Could you check a few things on this model? Use its own coordinates, in mm. Face numbers are marked on the shaded views. A direction names the side the tool comes from. Give positions to 0.01 mm unless a question says otherwise; leave off trailing zeros. Loops run counter-clockwise (first coordinate to the right, second up) from the corner with the lowest first, then second, coordinate; pieces in that order, holes last. Notation, with made-up numbers: M 60.25,54.5 L 65.25,54.5 A31 cw 65.25,88.5 Z; hole C -35,-33.75 d5. An arc over 180 degrees is marked long. Answer in a Markdown table with one row per item. Add a question column.
1. Which directions (+Z, -Z, +X, -X, +Y, -Y) give clear straight access to the entire face, cutting with the end or side of a thin tool? Please do the marked faces 3, 4, 5 and 6.
2. If we section it at D-D on y = -7.5: List the corners of the cut face in (x, z) for me.
3. Thinking about a two-plate mould opening in X: for the marked faces 1 and 2, which applies, released by +X, released by -X, zero draft, split by the parting line, or undercut?
4. I need wall thicknesses on line 1 along Y through (x, z) = (0, 11); line 2 along X through (y, z) = (19, 3.75); line 3 along X through (y, z) = (22.5, 10). Which ranges of each line are inside material? Lowest first, please. Write a range as from..to.
5. I'm going to push flat-ended pins straight in: pin 1 Ø2 at (y, z) = (-10, 11.5) entering from -X; pin 2 Ø4.5 at (x, y) = (-10.11, -10.45) entering from +Z; pin 3 Ø0.8 at (x, y) = (33, 0) entering from -Z. Where does each tip first touch, or does it pass through?
6. If we section it at A-A on z = 14.5: List the corners of the cut face in (x, y) for me, then the cut area to 3 significant figures.
7. If we section it at B-B on y = 0: Count the separate pieces of the cut face and the enclosed holes in it, then the cut area to 3 significant figures.
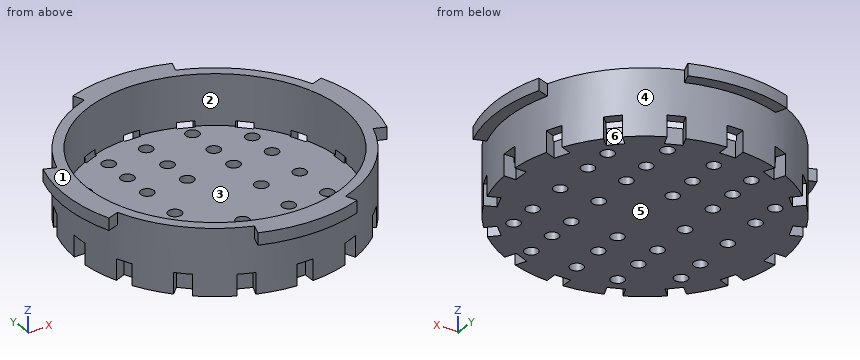
```python
from build123d import *

# Parameters (mm, degrees)
F0_R     = 34.25
F0_R_2   = 31.75
F1_DEPTH = 16.5
F2_R     = 34.25
F2_R_2   = 31.75
F3_DEPTH = 4
F5_DEPTH = 5.25
F7_D     = 3.3
F9_DEPTH = 3


with BuildPart() as f1:
    # F0 (on Top) → F1 (new body)
    with BuildSketch(Plane.XY):
        Circle(F0_R)
        Circle(F0_R_2, mode=Mode.SUBTRACT)
    extrude(amount=F1_DEPTH)

    # F2 (on face) → F3 (join)
    with BuildSketch(Plane(origin=(0, 0, 0), x_dir=(1, 0, 0), z_dir=(0, 0, -1))):
        Circle(F2_R)
        Circle(F2_R_2, mode=Mode.SUBTRACT)
        Circle(F2_R_2)
    extrude(amount=-F3_DEPTH)

    # F4 (on face) → F5 (cut)
    with BuildSketch(Plane(origin=(0, 0, 0), x_dir=(1, 0, 0), z_dir=(0, 0, -1))):
        with BuildLine():
            ThreePointArc((25.5912946517, 22.762867527), (24.2184072556, 24.2184072556), (22.762867527, 25.5912946517))
            Line((22.762867527, 25.5912946517), (20.6828733497, 23.5113004745))
            Line((20.6828733497, 23.5113004745), (23.5113004745, 20.6828733497))
            Line((23.5113004745, 20.6828733497), (25.5912946517, 22.762867527))
        make_face()
        with BuildLine():
            ThreePointArc((14.9323010635, 30.8235118854), (13.1069075585, 31.6428739885), (11.2367829334, 32.3542456149))
            Line((11.2367829334, 32.3542456149), (10.1110981964, 29.6366022557))
            Line((10.1110981964, 29.6366022557), (13.8066163264, 28.1058685262))
            Line((13.8066163264, 28.1058685262), (14.9323010635, 30.8235118854))
        make_face()
        with BuildLine():
            ThreePointArc((2, 34.1915559751), (0, 34.25), (-2, 34.1915559751))
            Line((-2, 34.1915559751), (-2, 31.25))
            Line((-2, 31.25), (2, 31.25))
            Line((2, 31.25), (2, 34.1915559751))
        make_face()
        with BuildLine():
            Line((-10.1110981964, 29.6366022557), (-11.2367829334, 32.3542456149))
            ThreePointArc((-11.2367829334, 32.3542456149), (-13.1069075585, 31.6428739885), (-14.9323010635, 30.8235118854))
            Line((-14.9323010635, 30.8235118854), (-13.8066163264, 28.1058685262))
            Line((-13.8066163264, 28.1058685262), (-10.1110981964, 29.6366022557))
        make_face()
        with BuildLine():
            Line((-20.6828733497, 23.5113004745), (-22.762867527, 25.5912946517))
            ThreePointArc((-22.762867527, 25.5912946517), (-24.2184072556, 24.2184072556), (-25.5912946517, 22.762867527))
            Line((-25.5912946517, 22.762867527), (-23.5113004745, 20.6828733497))
            Line((-23.5113004745, 20.6828733497), (-20.6828733497, 23.5113004745))
        make_face()
        with BuildLine():
            Line((-31.25, 2), (-34.1915559751, 2))
            ThreePointArc((-34.1915559751, 2), (-34.25, 0), (-34.1915559751, -2))
            Line((-34.1915559751, -2), (-31.25, -2))
            Line((-31.25, -2), (-31.25, 2))
        make_face()
        with BuildLine():
            Line((-29.6366022557, -10.1110981964), (-32.3542456149, -11.2367829334))
            ThreePointArc((-32.3542456149, -11.2367829334), (-31.6428739885, -13.1069075585), (-30.8235118854, -14.9323010635))
            Line((-30.8235118854, -14.9323010635), (-28.1058685262, -13.8066163264))
            Line((-28.1058685262, -13.8066163264), (-29.6366022557, -10.1110981964))
        make_face()
        with BuildLine():
            Line((-23.5113004745, -20.6828733497), (-25.5912946517, -22.762867527))
            ThreePointArc((-25.5912946517, -22.762867527), (-24.2184072556, -24.2184072556), (-22.762867527, -25.5912946517))
            Line((-22.762867527, -25.5912946517), (-20.6828733497, -23.5113004745))
            Line((-20.6828733497, -23.5113004745), (-23.5113004745, -20.6828733497))
        make_face()
        with BuildLine():
            Line((-13.8066163264, -28.1058685262), (-14.9323010635, -30.8235118854))
            ThreePointArc((-14.9323010635, -30.8235118854), (-13.1069075585, -31.6428739885), (-11.2367829334, -32.3542456149))
            Line((-11.2367829334, -32.3542456149), (-10.1110981964, -29.6366022557))
            Line((-10.1110981964, -29.6366022557), (-13.8066163264, -28.1058685262))
        make_face()
        with BuildLine():
            Line((-2, -31.25), (-2, -34.1915559751))
            ThreePointArc((-2, -34.1915559751), (0, -34.25), (2, -34.1915559751))
            Line((2, -34.1915559751), (2, -31.25))
            Line((2, -31.25), (-2, -31.25))
        make_face()
        with BuildLine():
            ThreePointArc((11.2367829334, -32.3542456149), (13.1069075585, -31.6428739885), (14.9323010635, -30.8235118854))
            Line((14.9323010635, -30.8235118854), (13.8066163264, -28.1058685262))
            Line((13.8066163264, -28.1058685262), (10.1110981964, -29.6366022557))
            Line((10.1110981964, -29.6366022557), (11.2367829334, -32.3542456149))
        make_face()
        with BuildLine():
            ThreePointArc((30.8235118854, -14.9323010635), (31.6428739885, -13.1069075585), (32.3542456149, -11.2367829334))
            Line((32.3542456149, -11.2367829334), (29.6366022557, -10.1110981964))
            Line((29.6366022557, -10.1110981964), (28.1058685262, -13.8066163264))
            Line((28.1058685262, -13.8066163264), (30.8235118854, -14.9323010635))
        make_face()
        with BuildLine():
            ThreePointArc((22.762867527, -25.5912946517), (24.2184072556, -24.2184072556), (25.5912946517, -22.762867527))
            Line((25.5912946517, -22.762867527), (23.5113004745, -20.6828733497))
            Line((23.5113004745, -20.6828733497), (20.6828733497, -23.5113004745))
            Line((20.6828733497, -23.5113004745), (22.762867527, -25.5912946517))
        make_face()
        with BuildLine():
            ThreePointArc((34.25, 0), (34.2353858759, 1.0004268719), (34.1915559751, 2))
            Line((34.1915559751, 2), (31.25, 2))
            Line((31.25, 2), (31.25, -2))
            Line((31.25, -2), (34.1915559751, -2))
            ThreePointArc((34.1915559751, -2), (34.2353858759, -1.0004268719), (34.25, 0))
        make_face()
        with BuildLine():
            ThreePointArc((32.3542456149, 11.2367829334), (31.6428739885, 13.1069075585), (30.8235118854, 14.9323010635))
            Line((30.8235118854, 14.9323010635), (28.1058685262, 13.8066163264))
            Line((28.1058685262, 13.8066163264), (29.6366022557, 10.1110981964))
            Line((29.6366022557, 10.1110981964), (32.3542456149, 11.2367829334))
        make_face()
        with BuildLine():
            Line((-28.1058685262, 13.8066163264), (-30.8235118854, 14.9323010635))
            ThreePointArc((-30.8235118854, 14.9323010635), (-31.6428739885, 13.1069075585), (-32.3542456149, 11.2367829334))
            Line((-32.3542456149, 11.2367829334), (-29.6366022557, 10.1110981964))
            Line((-29.6366022557, 10.1110981964), (-28.1058685262, 13.8066163264))
        make_face()
    extrude(amount=-F5_DEPTH, mode=Mode.SUBTRACT)

    # F7 (through all)
    with Locations(Plane(origin=(0, 0, 0), x_dir=(1, 0, 0), z_dir=(0, 0, -1))):
        with Locations((-10.1110981964, 0), (-10.1110981964, 10.4496451095), (-10.1110981964, 17.7097469568), (-20.8794418722, 17.7097469568), (-20.8794418722, 10.4496451095), (-20.8794418722, 0), (-20.8794418722, -10.5109745637), (-20.8794418722, -18.0052742362), (-10.1110981964, -25.1482781023), (-10.1110981964, -18.0052742362), (-10.1110981964, -10.5109745637), (0, -18.0052742362), (0, -10.5109745637), (0, -26.0850638151), (0, 10.4496451095), (0, 17.7097469568), (-10.1110981964, 25.5912946517), (11.6739207879, 25.5912946517), (0, 25.906637311), (11.6739207879, 17.7097469568), (11.6739207879, 10.4496451095), (11.6739207879, 0), (11.6739207879, -10.5109745637), (11.6739207879, -26.0850638151), (21.3930904865, -18.0052742362), (11.6739207879, -18.0052742362), (21.3930904865, -10.5109745637), (21.3930904865, 0), (21.3930904865, 10.4496451095), (21.3930904865, 17.7097469568)):
            Hole(F7_D / 2)

    # F8 (on face) → F9 (join)
    with BuildSketch(Plane.XY.offset(16.5)):
        with BuildLine():
            ThreePointArc((-32.2640173781, -11.4932885906), (-34.25, 0), (-32.2640173781, 11.4932885906))
            Line((-32.2640173781, 11.4932885906), (-35.0900626959, 12.5))
            ThreePointArc((-35.0900626959, 12.5), (-37.25, 0), (-35.0900626959, -12.5))
            Line((-35.0900626959, -12.5), (-32.2640173781, -11.4932885906))
        make_face()
        with BuildLine():
            Line((11.4932885906, 32.2640173781), (12.5, 35.0900626959))
            ThreePointArc((12.5, 35.0900626959), (0, 37.25), (-12.5, 35.0900626959))
            Line((-12.5, 35.0900626959), (-11.4932885906, 32.2640173781))
            ThreePointArc((-11.4932885906, 32.2640173781), (0, 34.25), (11.4932885906, 32.2640173781))
        make_face()
        with BuildLine():
            Line((35.0900626959, 12.5), (32.2640173781, 11.4932885906))
            ThreePointArc((32.2640173781, 11.4932885906), (33.7498525567, 5.8318052437), (34.25, 0))
            ThreePointArc((34.25, 0), (33.7498525567, -5.8318052437), (32.2640173781, -11.4932885906))
            Line((32.2640173781, -11.4932885906), (35.0900626959, -12.5))
            ThreePointArc((35.0900626959, -12.5), (37.25, 0), (35.0900626959, 12.5))
        make_face()
        with BuildLine():
            ThreePointArc((11.4932885906, -32.2640173781), (0, -34.25), (-11.4932885906, -32.2640173781))
            Line((-11.4932885906, -32.2640173781), (-12.5, -35.0900626959))
            ThreePointArc((-12.5, -35.0900626959), (0, -37.25), (12.5, -35.0900626959))
            Line((12.5, -35.0900626959), (11.4932885906, -32.2640173781))
        make_face()
    extrude(amount=-F9_DEPTH)


solid = f1.part
```
Results:
| question | item | result |
|---|---|---|
| 1 | face 3 | +Z |
| 1 | face 4 | -Z |
| 1 | face 5 | -Z, +X, -X, +Y, -Y |
| 1 | face 6 | +Z, -Z |
| 2 | outline | M -36.49,13.5 L -33.42,13.5 L -33.42,0 L 33.42,0 L 33.42,13.5 L 36.49,13.5 L 36.49,16.5 L 30.85,16.5 L 30.85,4 L -30.85,4 L -30.85,16.5 L -36.49,16.5 Z |
| 3 | face 1 | zero draft |
| 3 | face 2 | undercut |
| 4 | line 1 | -34.25..-31.75, 31.75..34.25 |
| 4 | line 2 | -28.5..-22.2, -19.56..-11.43, -8.79..-1.32, 1.32..10.36, 12.99..20.08, 22.71..28.5 |
| 4 | line 3 | -25.82..-22.4, 22.4..25.82 |
| 5 | pin 1 | x = -33.05 |
| 5 | pin 2 | z = 4 |
| 5 | pin 3 | z = 5.25 |
| 6 | outline | M -35.09,-12.5 L -32.26,-11.49 A34.25 ccw -11.49,-32.26 L -12.5,-35.09 A37.25 ccw 12.5,-35.09 L 11.49,-32.26 A34.25 ccw 32.26,-11.49 L 35.09,-12.5 A37.25 ccw 35.09,12.5 L 32.26,11.49 A34.25 ccw 11.49,32.26 L 12.5,35.09 A37.25 ccw -12.5,35.09 L -11.49,32.26 A34.25 ccw -32.26,11.49 L -35.09,12.5 A37.25 ccw Z; hole C 0,0 d63.5 |
| 6 | area | 812 mm2 |
| 7 | separate pieces | 7 |
| 7 | enclosed holes | 0 |
| 7 | area | 271 mm2 |
